Verification items for the finished model (mm, model axes). A direction names the side the tool comes from. Round coordinates to 2 decimals unless told otherwise and drop trailing zeros. Write each loop counter-clockwise with the first axis right and the second up, starting at its lowest first coordinate (ties: lowest second). Pieces come first, ordered by that corner, then holes. Notation, with made-up numbers: (28.25, -33) -> (41.25, -33) arc R5 cw to (41.25, -28) -> close; hole circle Ø7 at (2, 20). An arc over 180 degrees is marked (long way). Use CSV: the item, a comma, the result in double quotes.
```python
from build123d import *

# Parameters (mm, degrees)
F0_R     = 10
F1_DEPTH = 18
F3_DEPTH = 15
F4_R     = 5
F5_DEPTH = 3
F6_R     = 10
F6_R_2   = 5
F7_DEPTH = 15


with BuildPart() as f1:
    # F0 (on Top) → F1 (new body)
    with BuildSketch(Plane.XY):
        Circle(F0_R)
    extrude(amount=F1_DEPTH)

    # F2 (on face) → F3 (cut)
    with BuildSketch(Plane(origin=(0, 0, 0), x_dir=(1, 0, 0), z_dir=(0, 0, -1))):
        with BuildLine():
            Line((3.5, -3.5707142143), (3.5, 3.5707142143))
            ThreePointArc((3.5, 3.5707142143), (2.87748668, 4.0890182693), (2.1794494718, 4.5))
            Line((2.1794494718, 4.5), (-2.1794494718, 4.5))
            ThreePointArc((-2.1794494718, 4.5), (-2.87748668, 4.0890182693), (-3.5, 3.5707142143))
            Line((-3.5, 3.5707142143), (-3.5, -3.5707142143))
            ThreePointArc((-3.5, -3.5707142143), (-2.87748668, -4.0890182693), (-2.1794494718, -4.5))
            Line((-2.1794494718, -4.5), (2.1794494718, -4.5))
            ThreePointArc((2.1794494718, -4.5), (2.87748668, -4.0890182693), (3.5, -3.5707142143))
        make_face()
    extrude(amount=-F3_DEPTH, mode=Mode.SUBTRACT)

    # F4 (on face) → F5 (cut)
    with BuildSketch(Plane.XY.offset(18)):
        Circle(F4_R)
    extrude(amount=-F5_DEPTH, mode=Mode.SUBTRACT)

    # F6 (on face) → F7 (join)
    with BuildSketch(Plane.XY.offset(18)):
        Circle(F6_R)
        Circle(F6_R_2, mode=Mode.SUBTRACT)
        Circle(F6_R_2)
        with BuildLine():
            ThreePointArc((2, 2.2360679775), (2.7386127875, 1.2247448714), (3, 0))
            ThreePointArc((3, 0), (2.7386127875, -1.2247448714), (2, -2.2360679775))
            Line((2, -2.2360679775), (2, -3))
            Line((2, -3), (0, -3))
            Line((0, -3), (-2, -3))
            Line((-2, -3), (-2, -2.2360679775))
            ThreePointArc((-2, -2.2360679775), (-3, 0), (-2, 2.2360679775))
            Line((-2, 2.2360679775), (-2, 3))
            Line((-2, 3), (0, 3))
            Line((0, 3), (2, 3))
            Line((2, 3), (2, 2.2360679775))
        make_face(mode=Mode.SUBTRACT)
        with BuildLine():
            ThreePointArc((2, -2.2360679775), (2.7386127875, -1.2247448714), (3, 0))
            ThreePointArc((3, 0), (2.7386127875, 1.2247448714), (2, 2.2360679775))
            Line((2, 2.2360679775), (2, -2.2360679775))
        make_face()
        with BuildLine():
            Line((2, -3), (2, -2.2360679775))
            ThreePointArc((2, -2.2360679775), (1.0704662693, -2.8025170769), (0, -3))
            Line((0, -3), (2, -3))
        make_face()
        with BuildLine():
            Line((-2, -3), (0, -3))
            ThreePointArc((0, -3), (-1.0704662693, -2.8025170769), (-2, -2.2360679775))
            Line((-2, -2.2360679775), (-2, -3))
        make_face()
        with BuildLine():
            Line((-2, -2.2360679775), (-2, 2.2360679775))
            ThreePointArc((-2, 2.2360679775), (-3, 0), (-2, -2.2360679775))
        make_face()
        with BuildLine():
            ThreePointArc((-2, 2.2360679775), (-1.0704662693, 2.8025170769), (0, 3))
            Line((0, 3), (-2, 3))
            Line((-2, 3), (-2, 2.2360679775))
        make_face()
        with BuildLine():
            ThreePointArc((0, 3), (1.0704662693, 2.8025170769), (2, 2.2360679775))
            Line((2, 2.2360679775), (2, 3))
            Line((2, 3), (0, 3))
        make_face()
    extrude(amount=F7_DEPTH)


solid = f1.part
```
Q1. Mould release check, pull along X, two halves, no side actions. Record for faces 1 (the flat face through (-4, 0, 15)), 2 (the flat face through (-2.4, 0.1, 33)), 3 (the cylindrical face through (-2.17, -9.76, 16.27)): released by +X, released by -X, zero draft, split by the parting line, or undercut.
Filled in:
face 1,"undercut"
face 2,"zero draft"
face 3,"split by the parting line"
Q2. Go/stop test with flat-tipped pins: P1, Ø4, axis at y = -4.5, z = 14.5, coming from the +X side; P2, Ø3, axis at y = 6, z = 14.5, coming from the +X side; P3, Ø2, axis at y = -7, z = 15.5, coming from the +X side. Record where each tip stops, or that it passes through.
Filled in:
P1,"x = 9.68"
P2,"x = 8.93"
P3,"x = 8"
Q3. Section check C-C (z = 9). Record the cut outline in (x, y), plus the area to 3 significant figures.
Filled in:
outline,"circle Ø20 at (0, 0); hole (-3.5, -3.57) arc R5 ccw to (-2.18, -4.5) -> (2.18, -4.5) arc R5 ccw to (3.5, -3.57) -> (3.5, 3.57) arc R5 ccw to (2.18, 4.5) -> (-2.18, 4.5) arc R5 ccw to (-3.5, 3.57) -> close"
area,"253 mm²"
Q4. Access from +Z, -Z, +X, -X, +Y, -Y to the whole of each face (thin tool, end or side, straight path). Record for faces 4 (the flat face through (-3.5, 0, 7)), 5 (the flat face through (2, 0, 25)), 6 (the flat face through (4, 0, 15)).
Filled in:
face 4,"-Z"
face 5,"+Z, -Z"
face 6,"none"
Q5. Material ranges on L1, parallel to Y at x = 0, z = 17.3; L2, parallel to Z at x = -4.75, y = 0; L3, parallel to X at y = -2, z = 26, recorded low to high.
Filled in:
L1,"-10 to -5, 5 to 10"
L2,"0 to 15, 18 to 33"
L3,"-9.8 to -2, 2 to 9.8"
Q6. Section check D-D (x = -4). Record the cut outline in (y, z), plus the area to 3 significant figures.
Filled in:
outline,"(-9.17, 0) -> (9.17, 0) -> (9.17, 33) -> (-9.17, 33) -> close; hole (-3, 15) -> (3, 15) -> (3, 18) -> (-3, 18) -> close"
area,"587 mm²"
Q7. Section check A-A (y = 0). Record the cut outline in (x, z).
Filled in:
outline,"(-10, 0) -> (-3.5, 0) -> (-3.5, 15) -> (-5, 15) -> (-5, 18) -> (-2, 18) -> (-2, 33) -> (-10, 33) -> close; (2, 18) -> (5, 18) -> (5, 15) -> (3.5, 15) -> (3.5, 0) -> (10, 0) -> (10, 33) -> (2, 33) -> close"
Q8. Section check B-B (x = 1.5). Record the cut outline in (y, z).
Filled in:
outline,"(-9.89, 0) -> (-4.5, 0) -> (-4.5, 15) -> (-4.77, 15) -> (-4.77, 18) -> (-2.6, 18) -> (-2.6, 33) -> (-9.89, 33) -> close; (2.6, 18) -> (4.77, 18) -> (4.77, 15) -> (4.5, 15) -> (4.5, 0) -> (9.89, 0) -> (9.89, 33) -> (2.6, 33) -> close"
